```python
from build123d import *

# Parameters (mm, degrees)
SHEET_EXTRUDE_1_1_DEPTH = 100
THICKEN_1_T2            = 2
SHEET_METAL_1_DEPTH     = 100
SHEET_METAL_1_2_DEPTH   = 100


# Read off the part's stored shape, not the designer's step: Преобразовать-Твердое тело1
with BuildPart() as body_1:
    # Sheet Extrude 1: a surface, the sketch's curves swept straight by 100 mm
    with BuildLine(Plane.XY, mode=Mode.PRIVATE) as sheet_extrude_1_1_path:
        Line((-53.303838415, 0), (0, 0))
        Line((0, 0), (0, 66.585525728))
    sheet_extrude_1_1 = Shell.extrude(sheet_extrude_1_1_path.wire(), (0 * SHEET_EXTRUDE_1_1_DEPTH, 0 * SHEET_EXTRUDE_1_1_DEPTH, 1 * SHEET_EXTRUDE_1_1_DEPTH))
    add(Solid.thicken(sheet_extrude_1_1, -THICKEN_1_T2))

    # Sheet Metal 1 outline → Sheet Metal 1 (cut)
    with BuildSketch(Plane.XY):
        with BuildLine():
            Line((2, -2), (2, 1))
            ThreePointArc((2, 1), (1.121320344, -1.121320344), (-1, -2))
            Line((-1, -2), (2, -2))
        make_face()
    extrude(amount=SHEET_METAL_1_DEPTH, mode=Mode.SUBTRACT)

    # Sheet Metal 1 2 outline → Sheet Metal 1 2 (add)
    with BuildSketch(Plane.XY):
        with BuildLine():
            Line((0, 0), (0, 1))
            ThreePointArc((0, 1), (-0.292893219, 0.292893219), (-1, 0))
            Line((-1, 0), (0, 0))
        make_face()
    extrude(amount=SHEET_METAL_1_2_DEPTH)


solid = body_1.part
```
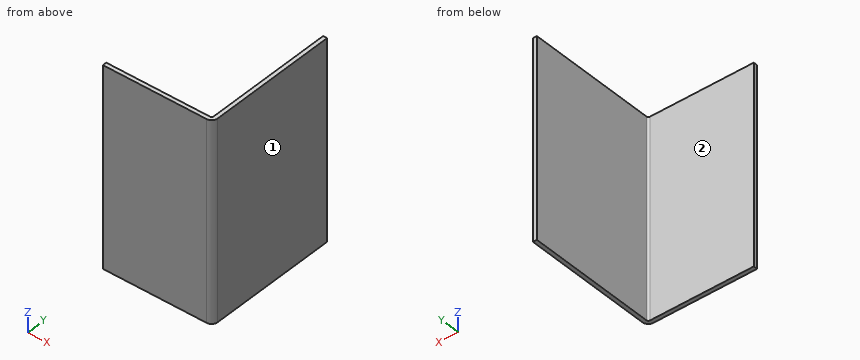
Geometry check sheet. Reference: the model listing, model coordinates, mm. Face numbers are marked on the shaded views. A direction names the side the tool comes from. Give positions to 0.01 mm unless a question says otherwise; leave off trailing zeros. Write each loop counter-clockwise with the first axis right and the second up, starting at its lowest first coordinate (ties: lowest second). Pieces come first, ordered by that corner, then holes. Notation, with made-up numbers: (40.25, 87.5) -> (63.25, 87.5) arc R21 cw to (63.25, 102.5) -> close; hole circle Ø2 at (10.5, -38.5). An arc over 180 degrees is marked (long way). One line per question, with ' | ' between items.
Item 1: Scan lines: line 1 along Y through (x, z) = (-41, 91); line 2 along X through (y, z) = (18.5, 59). Record each from-to range of solid material in increasing order.
Determined:
line 1: -2 to 0 | line 2: 0 to 2
Item 2: Depth check by flat-ended pin: pin 1 (8 mm diameter, centred on x = -24.5, z = 38, fed in from +Y); pin 2 (8 mm diameter, centred on y = 12.5, z = 84.5, fed in from -X). Enter the tip coordinate at first touch or a pass-through.
Determined:
pin 1: y = 0 | pin 2: x = 0
Item 3: Access from +Z, -Z, +X, -X, +Y, -Y to the whole of each face (thin tool, end or side, straight path). Record for the marked faces 1 and 2.
Determined:
face 1: +Z, -Z, +X, +Y, -Y | face 2: +Z, -Z, -X, +Y
Item 4: Sectioned sample at C-C, the plane x = -36. Record the boundary of the cut face in (y, z), plus the area to 3 significant figures.
Determined:
outline: (-2, 0) -> (0, 0) -> (0, 100) -> (-2, 100) -> close | area: 200 mm^2
Item 5: Sectioned sample at B-B, the plane y = 8. Record the boundary of the cut face in (x, z), plus the area to 3 significant figures.
Determined:
outline: (0, 0) -> (2, 0) -> (2, 100) -> (0, 100) -> close | area: 200 mm^2
Item 6: Sectioned sample at A-A, the plane z = 61. Record the boundary of the cut face in (x, y), plus the area to 3 significant figures.
Determined:
outline: (-53.3, -2) -> (-1, -2) arc R3 ccw to (2, 1) -> (2, 66.59) -> (0, 66.59) -> (0, 1) arc R1 cw to (-1, 0) -> (-53.3, 0) -> close | area: 242 mm^2
